```python
from build123d import *

# Parameters (mm, degrees)
F1_DEPTH = 63.5
F2_DEPTH = 25.4
F3_DEPTH = 7.9375
F5_R     = 6.35


# Not quite as in the source:
# - a feature names something its author has since deleted; it is built from what else it names


with BuildPart() as f1:
    # F0 (on Front) → F1 (new body, symmetric)
    with BuildSketch(Plane.XZ):
        Polygon((41.275, -9.525), (41.275, 9.525), (22.225, 9.525), (-41.275, 9.525), (-41.275, -9.525), align=None)
    extrude(amount=F1_DEPTH, both=True)

    # F0 (on Front) → F2 (join, symmetric)
    with BuildSketch(Plane.XZ):
        with BuildLine():
            Line((22.225, 9.525), (41.275, 9.525))
            Line((41.275, 9.525), (41.275, 46.0502))
            ThreePointArc((41.275, 46.0502), (45.9246798487, 57.2755201513), (57.15, 61.9252))
            Line((57.15, 61.9252), (60.325, 61.9252))
            Line((60.325, 61.9252), (60.325, 80.9752))
            Line((60.325, 80.9752), (57.15, 80.9752))
            add(Edge.make_bspline(
                [(46.42519144, 79.2877406183), (49.8648948299, 79.9027002695), (53.4381248944, 80.4666827005), (57.15, 80.9752)],
                knots=[116.6855453381, 116.6855453381, 116.6855453381, 116.6855453381, 121.6248811101, 121.6248811101, 121.6248811101, 121.6248811101], degree=3))
            ThreePointArc((46.42519144, 79.2877406183), (28.9159818308, 66.6073360608), (22.225, 46.0502))
            Line((22.225, 46.0502), (22.225, 9.525))
        make_face()
        Polygon((60.325, 80.9752), (60.325, 61.9252), (60.325, 57.15), (85.725, 57.15), (85.725, 80.9752), align=None)
    extrude(amount=F2_DEPTH, both=True)

    # F0 (on Front) → F3 (join, symmetric)
    with BuildSketch(Plane.XZ):
        with BuildLine():
            Line((-41.275, 9.525), (22.225, 9.525))
            Line((22.225, 9.525), (22.225, 46.0502))
            ThreePointArc((22.225, 46.0502), (28.9159818308, 66.6073360608), (46.42519144, 79.2877406183))
            add(Edge.make_bspline(
                [(-41.275, 9.525), (-41.5734088799, 21.7830526255), (-34.833440161, 64.760098527), (46.42519144, 79.2877406183)],
                knots=[0, 0, 0, 0, 116.6855453381, 116.6855453381, 116.6855453381, 116.6855453381], degree=3))
        make_face()
    extrude(amount=F3_DEPTH, both=True)

    # F0 (on Front) → F4 (revolve)
    with BuildSketch(Plane.XZ):
        Polygon((85.725, 80.9752), (85.725, 57.15), (111.125, 57.15), (111.125, 85.725), (85.725, 85.725), align=None)
    revolve(axis=Axis((85.725, 0, 71.4375), (0, 0, 1)))

    # F5
    f5_edges = [f1.edges().sort_by_distance(p)[0] for p in [
        (41.275, -63.5, 0),
        (-41.275, -63.5, 0),
        (-41.275, 63.5, 0),
        (41.275, 63.5, 0),
    ]]
    fillet(f5_edges, radius=F5_R)


solid = f1.part
```
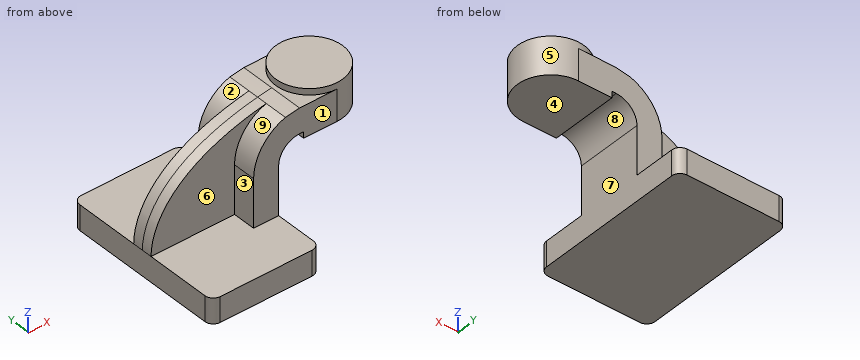
Read the model definition and answer for the solid it produces. Units are mm, in the model's axes. Face numbers are marked on the shaded views. A direction names the side the tool comes from. Coordinates: 2 decimals unless noted, no trailing zeros. Write each loop counter-clockwise with the first axis right and the second up, starting at its lowest first coordinate (ties: lowest second). Pieces come first, ordered by that corner, then holes. Notation, with made-up numbers: (22.25, 13.5) -> (58.25, 13.5) arc R30 cw to (58.25, 50.5) -> close; hole circle Ø6 at (86.5, 78.5). An arc over 180 degrees is marked (long way). Answer as a JSON object with one key per item and string values.
Q1. A tool of negligible diameter and unlimited length cuts with its end or side. For the marked faces 1, 2, 3, 4 and 5, from which of +Z, -Z, +X, -X, +Y, -Y can it reach the whole face along a straight path? Write none if from no direction.
The answers:
{"face 1": "+Z, +X, -X, -Y", "face 2": "+Z, -X, +Y", "face 3": "+Z, -X, -Y", "face 4": "-Z, +X, +Y, -Y", "face 5": "+Z"}
Q2. The part is cut by section D-D on x = 98. Give the vertices of the cut face in (y, z) (3 decimals).
The answers:
{"outline": "(-22.237, 57.15) -> (22.237, 57.15) -> (22.237, 85.725) -> (-22.237, 85.725) -> close"}
Q3. The part is cut by section B-B on y = 45. Give the vertices of the cut face in (x, z) (3 decimals).
The answers:
{"outline": "(-41.275, -9.525) -> (41.275, -9.525) -> (41.275, 9.525) -> (-41.275, 9.525) -> close"}
Q4. The part is cut by section A-A on z = 3.5. Give the vertices of the cut face in (x, y) (3 decimals), then the cut area to 3 significant figures.
The answers:
{"outline": "(-41.275, -57.15) arc R6.35 ccw to (-34.925, -63.5) -> (34.925, -63.5) arc R6.35 ccw to (41.275, -57.15) -> (41.275, 57.15) arc R6.35 ccw to (34.925, 63.5) -> (-34.925, 63.5) arc R6.35 ccw to (-41.275, 57.15) -> close", "area": "10,400 mm2"}
Q5. Flat-ended cylindrical pins translate along their axes: pin 1 Ø2.5 at (x, y) = (58, 7) entering from -Z; pin 2 Ø2.5 at (y, z) = (-4.5, 59.5) entering from -X; pin 3 Ø5 at (y, z) = (15, 34) entering from -X (3 decimals). Find the tip coordinate at first contact, or state that the pin passes through.
The answers:
{"pin 1": "stops at z = 61.92", "pin 2": "stops at x = -11.34", "pin 3": "stops at x = 22.225"}
Q6. Determine the mould class of the marked faces 6, 7, 8 and 9 for opening direction X: pulls with the +X half, pulls with the -X half, needs draft (parallel to the pull), parting line crosses it, or undercut.
The answers:
{"face 6": "needs draft", "face 7": "pulls with the +X half", "face 8": "undercut", "face 9": "pulls with the -X half"}
Q7. The part is cut by section C-C on x = 82. Give the vertices of the cut face in (y, z) (3 decimals), then the cut area to 3 significant figures.
The answers:
{"outline": "(-25.4, 57.15) -> (25.4, 57.15) -> (25.4, 80.975) -> (25.125, 80.975) -> (25.125, 85.725) -> (-25.125, 85.725) -> (-25.125, 80.975) -> (-25.4, 80.975) -> close", "area": "1,450 mm2"}
Q8. Consider line 1 (X direction, y = -53.5, z = 4.5) (3 decimals); line 2 (Z direction, x = 60, y = 22); line 3 (Z direction, x = 65.5, y = 13.5) (3 decimals). Determine where each line is inside the solid, lowest interval first. Write a range as [from, to].
The answers:
{"line 1": "x = [-41.275, 41.275]", "line 2": "z = [61.93, 80.98]", "line 3": "z = [57.15, 85.725]"}
